The listing builds one solid part. Answer for the finished solid, in the listing's coordinates (mm). Coordinates: 2 decimals unless noted, no trailing zeros. Loops run counter-clockwise (first coordinate to the right, second up) from the corner with the lowest first, then second, coordinate; pieces in that order, holes last. Notation, with made-up numbers: M -40,65.5 L -33,65.5 A22 ccw -33,104.5 Z; hole C 27.25,60.25 d4. An arc over 180 degrees is marked long. Return JSON: item names as keys, results as strings. Group by question number.
1. Straight lines are drawn through the part: L1, parallel to Y at x = 75, z = -11.5; L2, parallel to Y at x = -91, z = -16. For each, find the intervals that lie inside material, in ascending order. Write a range as from..to.
2. Section B-B (x = -101) is taken. Write down the section's boundary in (y, z).
3. Section A-A (z = -18.5) is taken. Write down the section's boundary in (x, y).
4. Given P1, Ø3, axis at x = -87.5, z = -11, coming from the -Y side; P2, Ø24, axis at x = 173, z = 9.5, coming from the -Y side; P3, Ø11, axis at x = 91, z = 13, coming from the -Y side, each flat-ended and moving along its own axis, determine where each tip first touches the part or whether it passes through.
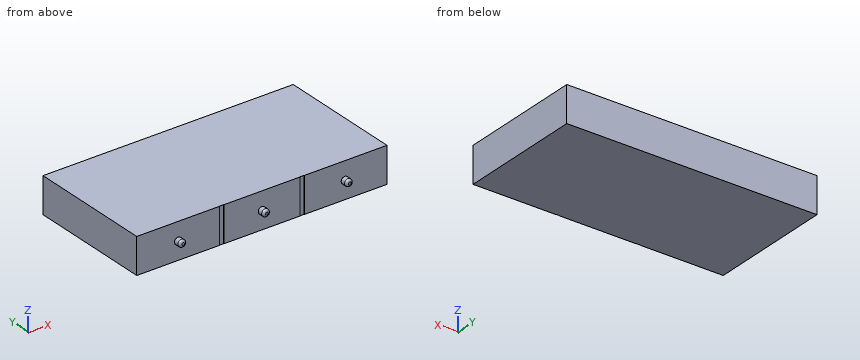
```python
from build123d import *

# Parameters (mm, degrees)
F0_W     = 560
F0_H     = 80
F1_DEPTH = 280
F2_W     = 10
F2_H     = 80
F3_DEPTH = 0.5
F4_R     = 8
F5_DEPTH = 15
F6_R     = 5


with BuildPart() as f1:
    # F0 (on Front) → F1 (new body)
    with BuildSketch(Plane.XZ):
        Rectangle(F0_W, F0_H)
    extrude(amount=F1_DEPTH)

    # F2 (on face) → F3 (cut)
    with BuildSketch(Plane.XZ.offset(280)):
        with Locations((-90, 0)):
            Rectangle(F2_W, F2_H)
        with Locations((90, 0)):
            Rectangle(F2_W, F2_H)
    extrude(amount=-F3_DEPTH, mode=Mode.SUBTRACT)

    # F4 (on face) → F5 (join)
    with BuildSketch(Plane.XZ.offset(280)):
        with Locations((-187.5, 0)):
            Circle(F4_R)
        Circle(F4_R)
        with Locations((185.5, 0)):
            Circle(F4_R)
    extrude(amount=F5_DEPTH)

    # F6
    f6_edges = [f1.edges().sort_by_distance(p)[0] for p in [
        (-195.5, -295, 0),
        (-8, -295, 0),
        (177.5, -295, 0),
    ]]
    fillet(f6_edges, radius=F6_R)


solid = f1.part
```
Worked out:
{
 "1": {"L1": "-280..0", "L2": "-279.5..0"},
 "2": {"outline": "M -280,-40 L 0,-40 L 0,40 L -280,40 Z"},
 "3": {"outline": "M -280,-280 L -95,-280 L -95,-279.5 L -85,-279.5 L -85,-280 L 85,-280 L 85,-279.5 L 95,-279.5 L 95,-280 L 280,-280 L 280,0 L -280,0 Z"},
 "4": {"P1": "y = -279.5", "P2": "y = -294.95", "P3": "y = -280"}
}
